from build123d import *

# Parameters (mm, degrees)
CYLINDER003_R     = 2.75
CYLINDER003_DEPTH = 3.4
CYLINDER002_R     = 1.5
CYLINDER002_DEPTH = 5
CYLINDER001_R     = 2.75
CYLINDER001_DEPTH = 3.4
CYLINDER_R        = 1.5
CYLINDER_DEPTH    = 5
BOX_W             = 49
BOX_H             = 35
BOX_DEPTH         = 4


with BuildPart() as cylinder003:
    # Cylinder003 → Cylinder003 (new body)
    with BuildSketch(Plane.XY.offset(11.6)):
        Circle(CYLINDER003_R)
    extrude(amount=CYLINDER003_DEPTH)


with BuildPart() as fusion001:
    # Cylinder002 → Cylinder002 (new body)
    with BuildSketch(Plane.XY.offset(10)):
        Circle(CYLINDER002_R)
    extrude(amount=CYLINDER002_DEPTH)

    # Fusion001: union Cylinder003
    add(cylinder003.part)


with BuildPart() as fusion001_1:
    # Fusion001 placement: moved
    add(fusion001.part.moved(Location((39.5, 17.5, -10))))


with BuildPart() as cylinder001:
    # Cylinder001 → Cylinder001 (new body)
    with BuildSketch(Plane.XY.offset(11.6)):
        Circle(CYLINDER001_R)
    extrude(amount=CYLINDER001_DEPTH)


with BuildPart() as fusion:
    # Cylinder → Cylinder (new body)
    with BuildSketch(Plane.XY.offset(10)):
        Circle(CYLINDER_R)
    extrude(amount=CYLINDER_DEPTH)

    # Fusion: union Cylinder001
    add(cylinder001.part)


with BuildPart() as fusion_1:
    # Fusion placement: moved
    add(fusion.part.moved(Location((9.5, 17.5, -10))))


with BuildPart() as obj1:
    # Box → Box (new body)
    with BuildSketch(Plane.XY):
        with Locations((24.5, 17.5)):
            Rectangle(BOX_W, BOX_H)
    extrude(amount=BOX_DEPTH)

    # Cut: cut Fusion
    add(fusion_1.part, mode=Mode.SUBTRACT)

    # Cut001: cut Fusion001
    add(fusion001_1.part, mode=Mode.SUBTRACT)


solid = obj1.part
Work out the finished part from the listing and answer in its coordinate system (mm). A direction names the side the tool comes from. Coordinates: 2 decimals unless noted, no trailing zeros. Write each loop counter-clockwise with the first axis right and the second up, starting at its lowest first coordinate (ties: lowest second). Pieces come first, ordered by that corner, then holes. Notation, with made-up numbers: (-28, -39.5) - (-22, -39.5) arc R21 cw to (-22, -21.5) - close; hole circle Ø10 at (63, -14). An arc over 180 degrees is marked (long way). One line per question, with ' | ' between items.
1) Find section A-A, the plane x = 39.5. Determine the outline of the cut face in (y, z).
Checks:
outline: (0, 0) - (16, 0) - (16, 1.6) - (14.75, 1.6) - (14.75, 4) - (0, 4) - close; (19, 0) - (35, 0) - (35, 4) - (20.25, 4) - (20.25, 1.6) - (19, 1.6) - close
2) Find section B-B, the plane y = 17.5. Determine the outline of the cut face in (x, z).
Checks:
outline: (0, 0) - (8, 0) - (8, 1.6) - (6.75, 1.6) - (6.75, 4) - (0, 4) - close; (11, 0) - (38, 0) - (38, 1.6) - (36.75, 1.6) - (36.75, 4) - (12.25, 4) - (12.25, 1.6) - (11, 1.6) - close; (41, 0) - (49, 0) - (49, 4) - (42.25, 4) - (42.25, 1.6) - (41, 1.6) - close
3) Consider probe 1 along X at (y, z) = (17.5, 3.3); probe 2 along X at (y, z) = (17.5, 0.6); probe 3 along Y at (x, z) = (39.5, 0.7). Determine where each line is inside the solid, lowest interval first. Write a range as [from, to].
Checks:
probe 1: [0, 6.75], [12.25, 36.75], [42.25, 49] | probe 2: [0, 8], [11, 38], [41, 49] | probe 3: [0, 16], [19, 35]
4) For faces 5 (the face through (9.142, 20.227, 2.783)), 6 (the face through (0, 17, 2)), determine the directions among +Z, -Z, +X, -X, +Y, -Y from which every point of the face is accessible in a straight line to the end or side of a thin tool.
Checks:
face 5: +Z | face 6: +Z, -Z, -X, +Y, -Y
5) Find section C-C, the plane z = 2.35. Determine the outline of the cut face in (x, y).
Checks:
outline: (0, 0) - (49, 0) - (49, 35) - (0, 35) - close; hole circle Ø5.5 at (9.5, 17.5); hole circle Ø5.5 at (39.5, 17.5)
6) The mould has two halves that part along Y. Classify faces 1 (the face through (24, 18, 0)), 2 (the face through (24, 35, 2)), 3 (the face through (24, 0, 2)), 4 (the face through (36.753, 17.621, 2.783)): +Y half, -Y half, draft (parallel to the pull), parting line (faces both ways), or undercut.
Checks:
face 1: draft | face 2: +Y half | face 3: -Y half | face 4: undercut
